Model file for the job. Use its own axes, mm. A direction names the side the tool comes from. Give positions to 0.01 mm unless a question says otherwise; leave off trailing zeros. Write each loop counter-clockwise with the first axis right and the second up, starting at its lowest first coordinate (ties: lowest second). Pieces come first, ordered by that corner, then holes.
```python
from build123d import *

# Parameters (mm, degrees)
BOSS_EXTRUDE1_DEPTH = 11.75


with BuildPart() as part:
    # Sketch1 → Boss-Extrude1 (new, symmetric)
    with BuildSketch(Plane.XY):
        with BuildLine():
            Line((-0.9, 2.170829335), (-0.9, 0.9))
            Line((-0.9, 0.9), (-2.170829335, 0.9))
            ThreePointArc((-2.170829335, 0.9), (-2.35, 0), (-2.170829335, -0.9))
            Line((-2.170829335, -0.9), (-0.9, -0.9))
            Line((-0.9, -0.9), (-0.9, -2.170829335))
            ThreePointArc((-0.9, -2.170829335), (0, -2.35), (0.9, -2.170829335))
            Line((0.9, -2.170829335), (0.9, -0.9))
            Line((0.9, -0.9), (2.170829335, -0.9))
            ThreePointArc((2.170829335, -0.9), (2.35, 0), (2.170829335, 0.9))
            Line((2.170829335, 0.9), (0.9, 0.9))
            Line((0.9, 0.9), (0.9, 2.170829335))
            ThreePointArc((0.9, 2.170829335), (0, 2.35), (-0.9, 2.170829335))
        make_face()
    extrude(amount=BOSS_EXTRUDE1_DEPTH, both=True)


solid = part.part
```
1. Which spindle directions (+Z, -Z, +X, -X, +Y, -Y) get a long thin tool onto all of the face, cutting with end or side? Do faces 1 (the flat face through (2, 0.9, 0)), 2 (the flat face through (-2, -0.9, 0)), 3 (the flat face through (2, -0.9, 0)), 4 (the flat face through (-0.9, 2, 0)). Say none if no direction does.
Calculated:
face 1: +Z, -Z, +X, +Y
face 2: +Z, -Z, -X, -Y
face 3: +Z, -Z, +X, -Y
face 4: +Z, -Z, -X, +Y
2. Probe probe 1 along X at (y, z) = (-1, -7.75); probe 2 along X at (y, z) = (0.1, 5.75). List the from-to ranges inside material, lowest first.
Calculated:
probe 1: x = -0.9 to 0.9
probe 2: x = -2.35 to 2.35
3. Slice it at B-B, the plane y = 1.3. Write the cut outline in (x, z).
Calculated:
outline: (-0.9, -11.75) - (0.9, -11.75) - (0.9, 11.75) - (-0.9, 11.75) - close
4. Slice it at A-A, the plane z = -10. Write the cut outline in (x, y).
Calculated:
outline: (-2.17, -0.9) - (-0.9, -0.9) - (-0.9, -2.17) arc R2.35 ccw to (0.9, -2.17) - (0.9, -0.9) - (2.17, -0.9) arc R2.35 ccw to (2.17, 0.9) - (0.9, 0.9) - (0.9, 2.17) arc R2.35 ccw to (-0.9, 2.17) - (-0.9, 0.9) - (-2.17, 0.9) arc R2.35 ccw to start
5. Pin check, flat tips, straight feed: P1, Ø1.5, axis at y = -1, z = 2.5, coming from the -X side; P2, Ø0.6, axis at x = 1.5, z = 4.5, coming from the +Y side; P3, Ø0.6, axis at y = 1.5, z = -0.5, coming from the -X side. Stop position of each tip, or through.
Calculated:
P1: stops at x = -2.34
P2: stops at y = 0.9
P3: stops at x = -0.9
